Verification items for the finished model (mm, model axes). Face numbers are marked on the shaded views. A direction names the side the tool comes from. Coordinates: 2 decimals unless noted, no trailing zeros. Write each loop counter-clockwise with the first axis right and the second up, starting at its lowest first coordinate (ties: lowest second). Pieces come first, ordered by that corner, then holes. Notation, with made-up numbers: (-38, 34) - (-5, 34) arc R26 ccw to (-5, 59) - close; hole circle Ø6 at (-34.75, 15). An arc over 180 degrees is marked (long way). Use one line per item in the form item = value. Start each with the question number.
(1) Sectioned sample at B-B (z = -11). Record the cut outline in (x, y), and give its area (3 significant figures).
(2) Mould release check, pull along Z, two halves, no side actions. Record for the marked faces 1, 2, 3 and 4: released by +Z, released by -Z, zero draft, split by the parting line, or undercut.
(3) Material ranges on line 1 (X direction, y = 12, z = 10); line 2 (X direction, y = 88, z = 17.5), recorded low to high. Write a range as [from, to].
(4) Sectioned sample at C-C (y = 29.5). Record the cut outline in (x, z), and give its area (3 significant figures).
(5) Sectioned sample at A-A (x = 9). Record the cut outline in (y, z), and give its area (3 significant figures).
(6) Tool access check on the marked faces 5 and 6. Record the directions out of +Z, -Z, +X, -X, +Y, -Y that give a thin tool (end or side, any length) a straight path to the whole face; none if there is none.
from build123d import *

# Parameters (mm, degrees)
ESBO_O1_W                = 40
ESBO_O1_H                = 40
ESBO_O1_W_2              = 37.6
ESBO_O1_H_2              = 37.6
RESSALTO_EXTRUS_O1_DEPTH = 210
FILETE1_R                = 3


with BuildPart() as part:
    # Esboço1 → Ressalto-extrusão1 (new, symmetric)
    with BuildSketch(Plane(origin=(0, 0, 0), x_dir=(1, 0, 0), z_dir=(0, 1, 0))):
        Rectangle(ESBO_O1_W, ESBO_O1_H)
        Rectangle(ESBO_O1_W_2, ESBO_O1_H_2, mode=Mode.SUBTRACT)
    extrude(amount=RESSALTO_EXTRUS_O1_DEPTH, both=True)

    # Filete1
    filete1_edges = [part.edges().sort_by_distance(p)[0] for p in [
        (-18.8, 0, 18.8),
        (18.8, 0, 18.8),
        (18.8, 0, -18.8),
        (-18.8, 0, -18.8),
        (-20, 0, -20),
        (20, 0, -20),
        (20, 0, 20),
        (-20, 0, 20),
    ]]
    fillet(filete1_edges, radius=FILETE1_R)


solid = part.part
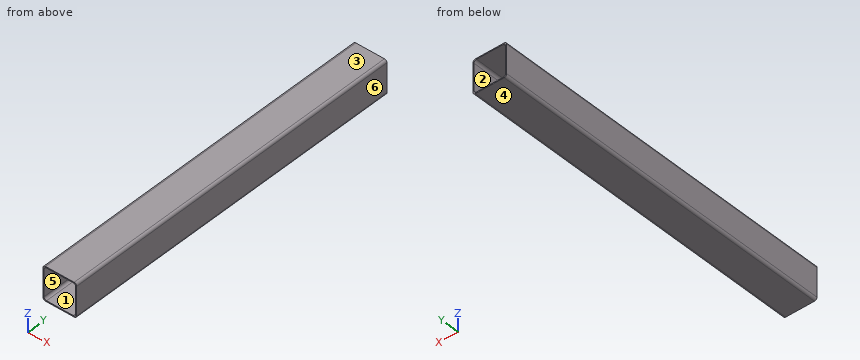
Answers below:
q1.outline = (-20, -210) - (-18.8, -210) - (-18.8, 210) - (-20, 210) - close; (18.8, -210) - (20, -210) - (20, 210) - (18.8, 210) - close
q1.area = 1,010 mm2
q2.face_1 = undercut
q2.face_2 = undercut
q2.face_3 = released by +Z
q2.face_4 = released by -Z
q3.line_1 = [-20, -18.8], [18.8, 20]
q3.line_2 = [-19.96, -18.27], [18.27, 19.96]
q4.outline = (-20, -17) arc R3 ccw to (-17, -20) - (17, -20) arc R3 ccw to (20, -17) - (20, 17) arc R3 ccw to (17, 20) - (-17, 20) arc R3 ccw to (-20, 17) - close; hole (-18.8, -15.8) arc R3 ccw to (-15.8, -18.8) - (15.8, -18.8) arc R3 ccw to (18.8, -15.8) - (18.8, 15.8) arc R3 ccw to (15.8, 18.8) - (-15.8, 18.8) arc R3 ccw to (-18.8, 15.8) - close
q4.area = 186 mm2
q5.outline = (-210, -20) - (210, -20) - (210, -18.8) - (-210, -18.8) - close; (-210, 18.8) - (210, 18.8) - (210, 20) - (-210, 20) - close
q5.area = 1,010 mm2
q6.face_5 = +Y, -Y
q6.face_6 = +Z, -Z, +X, +Y, -Y
